Job drawing, mm, ordinate dimensions from the low corner. One solid piece. A direction names the side the tool comes from. Give positions to 0.01 mm unless a question says otherwise; leave off trailing zeros. Order: outer loops, then holes, each group sorted by start corner. A loop starts at its lowest first (then second) coordinate and runs counter-clockwise, first axis right, second up.
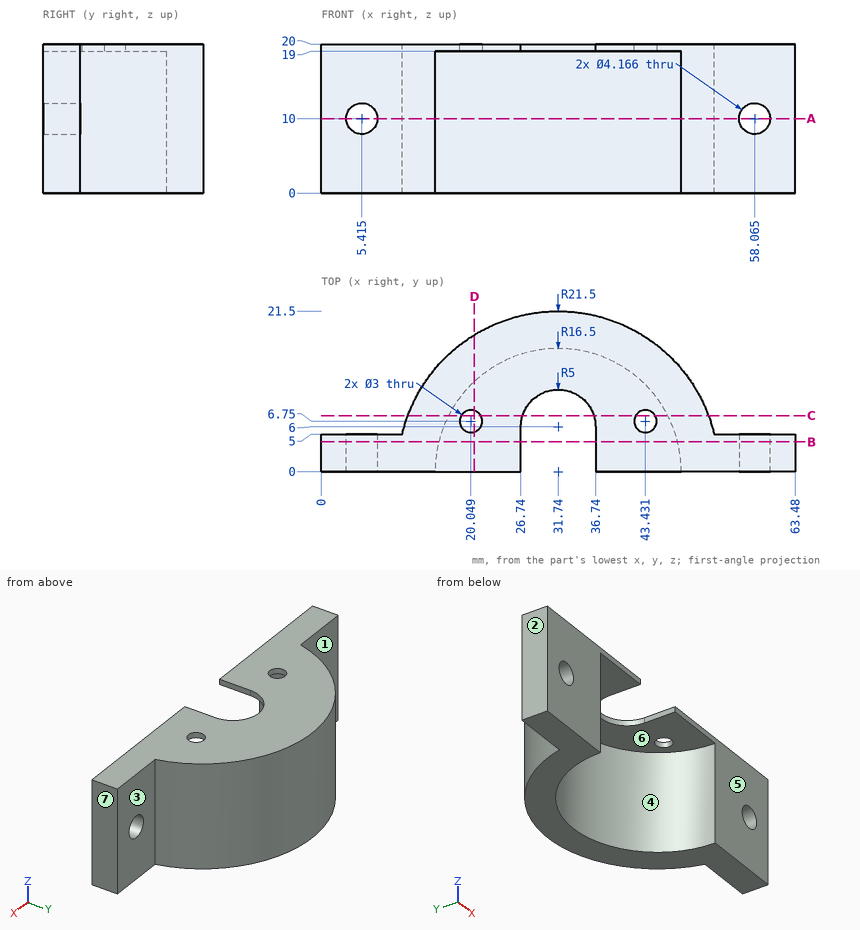
Item 1: Drill centre lines: probe 1 along Z at (x, y) = (23, 9.75); probe 2 along Y at (x, z) = (5.5, 2.25); probe 3 along X at (y, z) = (7, 5.5). Where is each one in solid material? Low to high.
Item 2: Band-saw the part on A-A on z = 10. List the corners of the cut face in (x, y), plus the area to 3 significant figures.
Item 3: Which spindle directions (+Z, -Z, +X, -X, +Y, -Y) get a long thin tool onto all of the face, cutting with end or side? Do the marked faces 1, 2 and 3. Say none if no direction does.
Item 4: Band-saw the part on C-C on y = 7.5. List the corners of the cut face in (x, z), plus the area to 3 significant figures.
Item 5: Pull direction X, two halves, no side cores. Call the marked faces 4, 5, 6 and 7: released by +X, released by -X, zero draft, split by the parting line, or undercut.
Item 6: Band-saw the part on B-B on y = 4. List the corners of the cut face in (x, z) (1 decimal), plus the area to 3 significant figures.
Item 7: Band-saw the part on D-D on x = 20.5. List the corners of the cut face in (y, z).
Item 8: Drop flat-ended pins along their axis: P1, Ø4, axis at y = 10, z = 8, coming from the -X side; P2, Ø3, axis at x = 7, z = 7.5, coming from the +Y side; P3, Ø4, axis at x = 39.5, y = 3, coming from the -Z side. Give the stop position or say it passes through.
Working result:
1. probe 1: z = 19 to 20
1. probe 2: y = 0 to 5
1. probe 3: x = 11.41 to 16.8, 46.68 to 52.07
2. outline: (0, 0) - (3.33, 0) - (3.33, 5) - (0, 5) - close; (7.5, 0) - (15.24, 0) arc R16.5 cw to (48.24, 0) - (55.98, 0) - (55.98, 5) - (52.65, 5) arc R21.5 ccw to (10.83, 5) - (7.5, 5) - close; (60.15, 0) - (63.48, 0) - (63.48, 5) - (60.15, 5) - close
2. area: 361 mm2
3. face 1: +Z, -Z, -X, +Y
3. face 2: +Z, -Z, -X, +Y, -Y
3. face 3: +Z, -Z, +X, +Y
4. outline: (11.59, 0) - (17.04, 0) - (17.04, 19) - (18.75, 19) - (18.75, 20) - (11.59, 20) - close; (21.35, 19) - (26.97, 19) - (26.97, 20) - (21.35, 20) - close; (36.51, 19) - (42.13, 19) - (42.13, 20) - (36.51, 20) - close; (44.73, 19) - (46.44, 19) - (46.44, 0) - (51.89, 0) - (51.89, 20) - (44.73, 20) - close
4. area: 233 mm2
5. face 4: undercut
5. face 5: zero draft
5. face 6: undercut
5. face 7: released by +X
6. outline: (0, 0) - (15.7, 0) - (15.7, 19) - (26.7, 19) - (26.7, 20) - (0, 20) - close; (36.7, 19) - (47.7, 19) - (47.7, 0) - (63.5, 0) - (63.5, 20) - (36.7, 20) - close; hole circle Ø4.2 at (5.4, 10); hole circle Ø4.2 at (58.1, 10)
6. area: 624 mm2
7. outline: (0, 19) - (5.32, 19) - (5.32, 20) - (0, 20) - close; (8.18, 19) - (12.08, 19) - (12.08, 0) - (18.33, 0) - (18.33, 20) - (8.18, 20) - close
8. P1: stops at x = 11.78
8. P2: stops at y = 5
8. P3: stops at z = 19
